For this review, use the dimensioned drawing (mm, ordinates from the lowest corner) and the shaded views. A direction names the side the tool comes from. Coordinates: 2 decimals unless noted, no trailing zeros. Loops run counter-clockwise (first coordinate to the right, second up) from the corner with the lowest first, then second, coordinate; pieces in that order, holes last. Notation, with made-up numbers: (68.25, 50) -> (107.25, 50) arc R32 ccw to (107.25, 87) -> close; hole circle Ø11 at (-21, 45.25). An arc over 180 degrees is marked (long way). Use one line per item in the form item = value. Start each with the question number.
1. Consider section B-B (x = 25). State the section outline as (y, z) points, then the cut area to 3 significant figures.
2. Consider section A-A (y = 6). State the section outline as (x, z) points, then the cut area to 3 significant figures.
3. Machinability: for the marked faces 4 and 5, which of the approach directions +Z, -Z, +X, -X, +Y, -Y give a long, thin tool a straight path to every point of the face, cutting with its end or side? Answer none if there is none.
4. Consider section D-D (x = 42.5). State the section outline as (y, z) points.
5. The part is to be moulded in two halves that separate along X. For the marked faces 1, 2 and 3, say which applies: released by +X, released by -X, zero draft, split by the parting line, or undercut.
6. For pin 1 (3 mm diameter, centred on x = 16.5, y = 21.5, fed in from -Z); pin 2 (2 mm diameter, centred on x = 26, y = 19, fed in from +Z), all flat-tipped, find the tip position at first contact; note any pin that passes through.
7. Wall thickness on line 1 (X direction, y = 22.5, z = 24); line 2 (Z direction, x = 29.5, y = 21.5): over which ranges is each line inside the solid? List them lowest first. Write a range as from..to.
8. Consider section C-C (z = 30). State the section outline as (x, y) points, then the cut area to 3 significant figures.
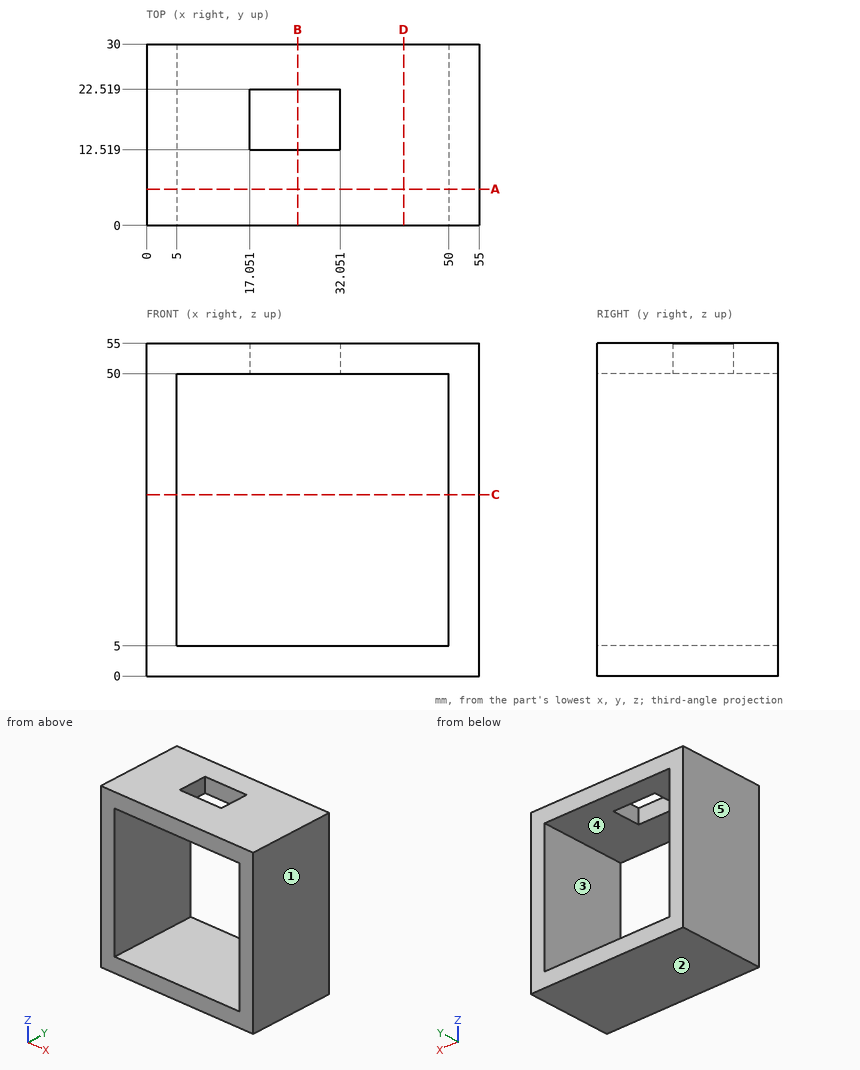
Geometry check:
q1.outline = (0, 0) -> (30, 0) -> (30, 5) -> (0, 5) -> close; (0, 50) -> (12.52, 50) -> (12.52, 55) -> (0, 55) -> close; (22.52, 50) -> (30, 50) -> (30, 55) -> (22.52, 55) -> close
q1.area = 250 mm²
q2.outline = (0, 0) -> (55, 0) -> (55, 55) -> (0, 55) -> close; hole (5, 5) -> (50, 5) -> (50, 50) -> (5, 50) -> close
q2.area = 1,000 mm²
q3.face_4 = +Y, -Y
q3.face_5 = +Z, -Z, -X, +Y, -Y
q4.outline = (0, 0) -> (30, 0) -> (30, 5) -> (0, 5) -> close; (0, 50) -> (30, 50) -> (30, 55) -> (0, 55) -> close
q5.face_1 = released by +X
q5.face_2 = zero draft
q5.face_3 = undercut
q6.pin_1 = 0
q6.pin_2 = 5
q7.line_1 = 0..5, 50..55
q7.line_2 = 0..5
q8.outline = (0, 0) -> (5, 0) -> (5, 30) -> (0, 30) -> close; (50, 0) -> (55, 0) -> (55, 30) -> (50, 30) -> close
q8.area = 300 mm²
